from build123d import *

# Parameters (mm, degrees)
SM_BASE_FLANGE_2_DEPTH   = 20
HOLE_WIZARD_M3_1_D       = 3.2
SKETCH_24_R              = 6.1
CUT_EXTRUDE_2_DEPTH      = 67.332495807
HOLE_WIZARD_M4_1_D       = 4.3
HOLE_WIZARD_M2_5_1_D     = 2.7
PATTERN_CIRCULAR_1_COUNT = 3


# Sheet-metal steps are written as plain solids
with BuildPart() as part:
    # 草圖16 → 基材-凸緣2 (new, symmetric)
    with BuildSketch(Plane.XY):
        with BuildLine():
            Line((36, 0), (0.7366, 0))
            ThreePointArc((0.7366, 0), (0.215745145, 0.215745145), (0, 0.7366))
            Line((0, 0.7366), (0, 48))
            Line((0, 48), (-4, 48))
            Line((-4, 48), (-4, 0.7366))
            ThreePointArc((-4, 0.7366), (-2.61268198, -2.61268198), (0.7366, -4))
            Line((0.7366, -4), (36, -4))
            Line((36, -4), (36, 0))
        make_face()
    extrude(amount=SM_BASE_FLANGE_2_DEPTH, both=True)

    # M3 餘隙孔1 (through all)
    with Locations(Plane(origin=(0, 0, 0), x_dir=(-1, 0, 0), z_dir=(0, 1, 0))):
        with Locations((-27, 17.5), (-11, 2.5), (-11, 17.5), (-27, 2.5)):
            Hole(HOLE_WIZARD_M3_1_D / 2)

    # 草圖24 → 除料-伸長2 (cut, through all)
    with BuildSketch(Plane.XZ.offset(4)):
        with Locations(Location((19, -10, 0), (0, 0, 270))):
            Circle(SKETCH_24_R)
    extrude(amount=-CUT_EXTRUDE_2_DEPTH, mode=Mode.SUBTRACT)

    # M4 餘隙孔1 (through all)
    with Locations(Plane(origin=(0, 0, 0), x_dir=(0, 0, 1), z_dir=(1, 0, 0))):
        with Locations((0, -44), (15, -44), (15, -24), (0, -24)):
            Hole(HOLE_WIZARD_M4_1_D / 2)

    # M2.5 餘隙孔1 (through all)
    with Locations(Plane(origin=(0, -4, 0), x_dir=(-1, 0, 0), z_dir=(0, -1, 0))):
        with Locations((-10.5, 10)):
            hole_wizard_m2_5_1 = Hole(HOLE_WIZARD_M2_5_1_D / 2)

    # 環狀複製排列1: M2.5 餘隙孔1 ×3 about axis
    pattern_circular_1_axis = Axis((19, 0, -10), (0, 1, 0))
    for i in range(1, PATTERN_CIRCULAR_1_COUNT):
        add(hole_wizard_m2_5_1.rotate(pattern_circular_1_axis, i * 360 / PATTERN_CIRCULAR_1_COUNT), mode=Mode.SUBTRACT)


solid = part.part
Geometry: final body of the model. Coordinates: model frame, mm. Coordinates: 2 decimals unless noted, no trailing zeros. Order: outer loops, then holes, each group sorted by start corner. A loop starts at its lowest first (then second) coordinate and runs counter-clockwise, first axis right, second up.
(1) Section query C-C (z = 6.5). Return the cut outline in (x, y), plus the area to 3 significant figures.
(2) Material intervals for probe 1 along X at (y, z) = (-2, -10); probe 2 along Z at (x, y) = (11, -3); probe 3 along X at (y, z) = (-2, 17), sorted ascending.
(3) Section query B-B (z = 0). Return the cut outline in (x, y), plus the area to 3 significant figures.
(4) First-contact query: pin 1 (8 mm diameter, centred on x = 6, z = 5, fed in from +Y); pin 2 (4 mm diameter, centred on y = 4.5, z = 6, fed in from +X). Flat tips, straight axial feed; report the tip coordinate or a pass-through.
(5) Draft query along Y for faces 1 (the face through (0, 24, -4)), 2 (the face through (-2.03, 26.1, 0.47)), 3 (the face through (19, 0, 0)). Return one class per face: pulls with the +Y half, pulls with the -Y half, needs draft (parallel to the pull), parting line crosses it, or undercut.
(6) Section query D-D (x = 10.5). Return the cut outline in (y, z).
(7) Section query A-A (x = 19). Return the cut outline in (y, z), plus the area to 3 significant figures.
Solution:
1. outline: (-4, 0.74) arc R4.74 ccw to (0.74, -4) - (36, -4) - (36, 0) - (0.74, 0) arc R0.74 cw to (0, 0.74) - (0, 48) - (-4, 48) - close
1. area: 347 mm2
2. probe 1: x = -3.13 to 9.15, 11.85 to 12.9, 25.1 to 36
2. probe 2: z = -20 to -11.25, -8.75 to 0.9, 4.1 to 15.9, 19.1 to 20
2. probe 3: x = -3.13 to 9.48, 12.52 to 25.48, 28.52 to 36
3. outline: (-4, 0.74) arc R4.74 ccw to (0.74, -4) - (36, -4) - (36, 0) - (0.74, 0) arc R0.74 cw to (0, 0.74) - (0, 21.85) - (-4, 21.85) - close; (-4, 26.15) - (0, 26.15) - (0, 41.85) - (-4, 41.85) - close; (-4, 46.15) - (0, 46.15) - (0, 48) - (-4, 48) - close
3. area: 313 mm2
4. pin 1: stops at y = 0
4. pin 2: stops at x = 0
5. face 1: needs draft
5. face 2: undercut
5. face 3: pulls with the +Y half
6. outline: (-4, -20) - (0, -20) - (0, -11.35) - (-4, -11.35) - close; (-4, -8.65) - (0, -8.65) - (0, 0.98) - (-4, 0.98) - close; (-4, 4.02) - (0, 4.02) - (0, 15.98) - (-4, 15.98) - close; (-4, 19.02) - (0, 19.02) - (0, 20) - (-4, 20) - close
7. outline: (-4, -20) - (0, -20) - (0, -16.1) - (-4, -16.1) - close; (-4, -3.9) - (0, -3.9) - (0, 20) - (-4, 20) - close
7. area: 111 mm2
